```python
from build123d import *

# Parameters (mm, degrees)
BOSS_EXTRUDE2_DEPTH = 6.35
CUT_EXTRUDE1_DEPTH  = 7.3500001
BOSS_EXTRUDE3_DEPTH = 6.35
SKETCH10_R          = 3.96875
CUT_EXTRUDE2_DEPTH  = 7.35
SKETCH11_R          = 9.525
CUT_EXTRUDE4_DEPTH  = 7.35
BOSS_EXTRUDE4_DEPTH = 6.35
SKETCH13_R          = 1.75
CUT_EXTRUDE5_DEPTH  = 7.35
LPATTERN1_COUNT     = 2
LPATTERN1_PITCH     = 64
SKETCH14_R          = 2.54
CUT_EXTRUDE6_DEPTH  = 7.35
SKETCH15_R          = 1.75
CUT_EXTRUDE7_DEPTH  = 7.35
SKETCH16_R          = 1.75
CUT_EXTRUDE8_DEPTH  = 7.35
SKETCH17_R          = 1.75
CUT_EXTRUDE9_DEPTH  = 7.35
SKETCH19_R          = 3.96875
CUT_EXTRUDE11_DEPTH = 7.35
SKETCH21_R          = 2.54
CUT_EXTRUDE12_DEPTH = 7.35
SKETCH22_R          = 3.175
CUT_EXTRUDE13_DEPTH = 7.35
SKETCH23_R          = 3.96875
CUT_EXTRUDE14_DEPTH = 7.35
SKETCH24_R          = 4.285761756
SKETCH24_R_2        = 5.640780493
BOSS_EXTRUDE5_DEPTH = 6.35
CUT_EXTRUDE15_DEPTH = 7.35
FILLET1_R           = 3.175


with BuildPart() as part:
    # Sketch6 → Boss-Extrude2 (new body)
    with BuildSketch(Plane.XY):
        with BuildLine():
            Line((-68.006850091, -76.67090114), (-109.486767671, -48.656527855))
            Line((-109.486767671, -48.656527855), (-118.371760678, -61.812230963))
            Line((-118.371760678, -61.812230963), (18.447551645, -154.216158235))
            Line((18.447551645, -154.216158235), (135.729459338, 19.43912279))
            Line((135.729459338, 19.43912279), (-1.089852986, 111.843050063))
            Line((-1.089852986, 111.843050063), (-73.946795643, 3.966284577))
            Line((-73.946795643, 3.966284577), (-56.624438948, -7.732749433))
            ThreePointArc((-56.624438948, -7.732749433), (-43.058385537, 37.577891571), (0, 57.15))
            ThreePointArc((0, 57.15), (56.404848571, 31.095576642), (70.829334649, -29.338471048))
            add(Edge.make_bspline(
                [(70.829334649, -29.338471048), (70.811686062, -29.418295928), (70.776015112, -29.578104383), (70.713320217, -29.85478305), (70.619021771, -30.262929245), (70.501052001, -30.762086912), (70.364034474, -31.322191481), (70.199318515, -31.970958926), (70.000453855, -32.723919765), (69.795103485, -33.469783355), (69.582015398, -34.214296028), (69.361377803, -34.956693289), (69.133257682, -35.696762218), (68.838782679, -36.61892651), (68.470566207, -37.720710028), (68.019498024, -38.998776477), (67.474836154, -40.448808619), (66.901337925, -41.887676852), (66.299328392, -43.31485223), (65.669141732, -44.729810424), (65.011119088, -46.132040323), (64.325609411, -47.52103904), (63.612968547, -48.896314904), (62.87355937, -50.257385735), (62.107751613, -51.603779381), (61.315921169, -52.935034173), (60.49845004, -54.250698756), (59.655726138, -55.550331897), (58.571247582, -57.154294757), (57.220953058, -59.045283389), (55.576035723, -61.200397094), (53.604026134, -63.590264702), (51.54329346, -65.904053004), (49.39728314, -68.138962994), (47.169496434, -70.29235602), (44.863486103, -72.361752995), (42.482847363, -74.344831806), (40.031215607, -76.239428526), (36.882516177, -78.494556171), (32.976808929, -81.016011003), (28.250788286, -83.68089187), (21.41551215, -86.919136497), (14.30829026, -89.526654921), (6.996956895, -91.488176442), (-0.451922312, -92.797413176), (-6.61686174, -93.456358442), (-12.81195397, -93.702029749), (-19.009644204, -93.537285056), (-25.183124422, -92.966685286), (-31.306438312, -91.996382122), (-36.598524037, -90.804323442), (-41.072542301, -89.543185606), (-44.752319298, -88.33589156), (-47.664184976, -87.27761875), (-50.541347258, -86.128353728), (-53.381128552, -84.889612663), (-56.180924218, -83.562977818), (-58.593536599, -82.326710176), (-60.633378351, -81.214215821), (-62.313751085, -80.252471782), (-63.646071553, -79.462491566), (-64.966093336, -78.652178853), (-66.222359154, -77.854259082), (-67.143044791, -77.250601571), (-67.736251212, -76.85365602), (-68.006850091, -76.67090114)],
                knots=[0.071020771, 0.071020771, 0.071020771, 0.071020771, 0.071020771, 0.072848477, 0.074676184, 0.07650389, 0.078331597, 0.08198701, 0.085642423, 0.089297836, 0.092953249, 0.096608662, 0.100264075, 0.103919488, 0.107574901, 0.114885727, 0.122196554, 0.12950738, 0.136818214, 0.144129048, 0.151439882, 0.158750716, 0.166061558, 0.173372401, 0.180683243, 0.187994085, 0.195304924, 0.202615763, 0.209926602, 0.217237441, 0.231859103, 0.246480766, 0.261102426, 0.275724085, 0.290345754, 0.304967424, 0.319589099, 0.334210774, 0.348832457, 0.36345414, 0.392697464, 0.421940789, 0.451184112, 0.506140643, 0.535383973, 0.564627303, 0.593870641, 0.623113979, 0.652357319, 0.68160066, 0.710843985, 0.740087309, 0.754708984, 0.769330659, 0.783952333, 0.798574008, 0.813195669, 0.82781733, 0.842438991, 0.849749821, 0.857060652, 0.86437149, 0.871682327, 0.878993165, 0.885158103, 0.885158103, 0.885158103, 0.885158103, 0.885158103], degree=4))
        make_face()
    extrude(amount=BOSS_EXTRUDE2_DEPTH)

    # Sketch8 → Cut-Extrude1 (cut, through all)
    with BuildSketch(Plane.XY.offset(6.35)):
        Polygon((-71.011229489, -93.798205788), (-53.378672597, -90.381637707), (-42.854110111, -97.489632113), (-39.43754203, -115.122189004), align=None)
    extrude(amount=-CUT_EXTRUDE1_DEPTH, mode=Mode.SUBTRACT)

    # Sketch9 → Boss-Extrude3 (add, through all)
    with BuildSketch(Plane.XY.offset(6.35)):
        Polygon((-1.089852986, 111.843050063), (-109.486767671, -48.656527855), (27.332544652, -141.060455127), (135.729459338, 19.43912279), align=None)
    extrude(amount=-BOSS_EXTRUDE3_DEPTH)

    # Sketch10 → Cut-Extrude2 (cut, through all)
    with BuildSketch(Plane.XY.offset(6.35)):
        with Locations((4.996496209, -84.796642912)):
            Circle(SKETCH10_R)
        with Locations((40.816310536, -31.759477627)):
            Circle(SKETCH10_R)
        with Locations((76.636124864, 21.277687659)):
            Circle(SKETCH10_R)
        with Locations((-45.295165913, -45.214466102)):
            Circle(SKETCH10_R)
    extrude(amount=-CUT_EXTRUDE2_DEPTH, mode=Mode.SUBTRACT)

    # Sketch11 → Cut-Extrude4 (cut, through all)
    with BuildSketch(Plane.XY.offset(6.35)):
        Circle(SKETCH11_R)
    extrude(amount=-CUT_EXTRUDE4_DEPTH, mode=Mode.SUBTRACT)

    # Sketch12 → Boss-Extrude4 (add, through all)
    with BuildSketch(Plane.XY.offset(6.35)):
        Polygon((135.729459338, 19.43912279), (67.319803176, 65.641086427), (88.643786393, 97.214773886), (157.053442554, 51.01281025), align=None)
    extrude(amount=-BOSS_EXTRUDE4_DEPTH)

    # Sketch13 → Cut-Extrude5 (cut, through all)
    with BuildSketch(Plane.XY.offset(6.35)):
        with Locations((94.899221836, -29.671127724)):
            Circle(SKETCH13_R)
    cut_extrude5 = extrude(amount=-CUT_EXTRUDE5_DEPTH, mode=Mode.SUBTRACT)

    # LPattern1: Cut-Extrude5 ×2
    with Locations(*[Vector(-0.559684599, -0.828705708, 0) * (i * LPATTERN1_PITCH) for i in range(1, LPATTERN1_COUNT)]):
        add(cut_extrude5, mode=Mode.SUBTRACT)

    # Sketch14 → Cut-Extrude6 (cut, through all)
    with BuildSketch(Plane.XY.offset(6.35)):
        with Locations((71.72703343, -52.635713164)):
            Circle(SKETCH14_R)
        with Locations((35.907219102, -105.67287845)):
            Circle(SKETCH14_R)
        with Locations((115.740620068, 63.589229581)):
            Circle(SKETCH14_R)
    extrude(amount=-CUT_EXTRUDE6_DEPTH, mode=Mode.SUBTRACT)

    # Sketch15 → Cut-Extrude7 (cut, through all)
    with BuildSketch(Plane.XY.offset(6.35)):
        with Locations((-105.147343009, -59.249804902)):
            Circle(SKETCH15_R)
        with Locations((15.885125585, -140.991740566)):
            Circle(SKETCH15_R)
        with Locations((1.472573075, 98.618632394)):
            Circle(SKETCH15_R)
    extrude(amount=-CUT_EXTRUDE7_DEPTH, mode=Mode.SUBTRACT)

    # Sketch16 → Cut-Extrude8 (cut, through all)
    with BuildSketch(Plane.XY.offset(6.35)):
        with Locations((92.060354474, 79.582216994)):
            Circle(SKETCH16_R)
        with Locations((139.420885662, 47.596242169)):
            Circle(SKETCH16_R)
    extrude(amount=-CUT_EXTRUDE8_DEPTH, mode=Mode.SUBTRACT)

    # Sketch17 → Cut-Extrude9 (cut, through all)
    with BuildSketch(Plane.XY.offset(6.35)):
        with Locations((-26.311406216, 17.769986014)):
            Circle(SKETCH17_R)
        with Locations((17.769986014, 26.311406216)):
            Circle(SKETCH17_R)
    extrude(amount=-CUT_EXTRUDE9_DEPTH, mode=Mode.SUBTRACT)

    # Sketch19 → Cut-Extrude11 (cut, through all)
    with BuildSketch(Plane.XY.offset(6.35)):
        with Locations((-65.680233685, -85.904783923)):
            Circle(SKETCH19_R)
    extrude(amount=-CUT_EXTRUDE11_DEPTH, mode=Mode.SUBTRACT)

    # Sketch21 → Cut-Extrude12 (cut, through all)
    with BuildSketch(Plane.XY.offset(6.35)):
        with Locations((-13.666272317, 70.530227577)):
            Circle(SKETCH21_R)
        with Locations((26.00698069, 78.217505758)):
            Circle(SKETCH21_R)
        with Locations((-86.729358658, -71.688795112)):
            Circle(SKETCH21_R)
        with Locations((-8.64928203, -120.590613931)):
            Circle(SKETCH21_R)
    extrude(amount=-CUT_EXTRUDE12_DEPTH, mode=Mode.SUBTRACT)

    # Sketch22 → Cut-Extrude13 (cut, through all)
    with BuildSketch(Plane.XY.offset(6.35)):
        with Locations((-26.311406216, 17.769986014)):
            Circle(SKETCH22_R)
        with Locations((17.769986014, 26.311406216)):
            Circle(SKETCH22_R)
    extrude(amount=-CUT_EXTRUDE13_DEPTH, mode=Mode.SUBTRACT)

    # Sketch23 → Cut-Extrude14 (cut, through all)
    with BuildSketch(Plane.XY.offset(6.35)):
        with Locations((-105.147343009, -59.249804902)):
            Circle(SKETCH23_R)
    extrude(amount=-CUT_EXTRUDE14_DEPTH, mode=Mode.SUBTRACT)

    # Sketch24 → Boss-Extrude5 (add, through all)
    with BuildSketch(Plane.XY.offset(6.35)):
        with Locations((-86.729358658, -71.688795112)):
            Circle(SKETCH24_R)
        with Locations((-65.680233685, -85.904783923)):
            Circle(SKETCH24_R_2)
    extrude(amount=-BOSS_EXTRUDE5_DEPTH)

    # Sketch25 → Cut-Extrude15 (cut, through all)
    with BuildSketch(Plane.XY.offset(6.35)):
        Polygon((85.800588631, 93.004948891), (87.167215863, 85.951926135), (71.529628171, 62.797888664), (67.319803176, 65.641086427), align=None)
    extrude(amount=-CUT_EXTRUDE15_DEPTH, mode=Mode.SUBTRACT)

    # Fillet1
    fillet1_edges = [part.edges().sort_by_distance(p)[0] for p in [
        (-1.089852986, 111.843050063, 3.175),
        (18.447551645, -154.216158235, 3.175),
        (-118.371760678, -61.812230963, 3.175),
        (85.800588631, 93.004948891, 3.175),
        (87.167215863, 85.951926135, 3.175),
        (71.529628171, 62.797888664, 3.175),
        (-39.43754203, -115.122189004, 3.175),
        (-71.011229489, -93.798205788, 3.175),
        (-53.378672597, -90.381637707, 3.175),
        (-42.854110111, -97.489632113, 3.175),
        (157.053442554, 51.01281025, 3.175),
        (88.643786393, 97.214773886, 3.175),
    ]]
    fillet(fillet1_edges, radius=FILLET1_R)


solid = part.part
```
The listing builds one solid part. Answer for the finished solid, in the listing's coordinates (mm). A direction names the side the tool comes from. Give positions to 0.01 mm unless a question says otherwise; leave off trailing zeros. Order: outer loops, then holes, each group sorted by start corner. A loop starts at its lowest first (then second) coordinate and runs counter-clockwise, first axis right, second up.
Item 1: For a pull along Y with two mould halves and no side action, classify faces 3 (the face through (-28.65, 19.92, 3.22)), 4 (the face through (-48.17, -93.9, 3.22)), 5 (the face through (21, -19, 6.35)) as pulls with the +Y half, pulls with the -Y half, needs draft (parallel to the pull), parting line crosses it, or undercut.
From the geometry:
face 3: undercut
face 4: pulls with the -Y half
face 5: needs draft
Item 2: Find the intervals of material crossed by probe 1 along X at (y, z) = (77, 3.25); probe 2 along X at (y, z) = (65.5, 4.5); probe 3 along Y at (x, z) = (0, 3.5) (3 decimals), in increasing order.
From the geometry:
probe 1: x = -24.62 to 23.78, 28.24 to 50.5, 81.12 to 118.58
probe 2: x = -32.39 to 67.53, 73.35 to 114.07, 117.41 to 135.6
probe 3: y = -141.757 to -9.525, 9.525 to 97.673, 99.564 to 110.601
Item 3: The part is cut by section C-C, the plane y = -72.5. Give the vertices of the cut face in (x, z).
From the geometry:
outline: (-102.55, 0) - (73.64, 0) - (73.64, 6.35) - (-102.55, 6.35) - close
Item 4: The part is cut by section A-A, the plane y = 0. Give the vertices of the cut face in (x, z) (3 decimals), and give its area (3 significant figures).
From the geometry:
outline: (-76.626, 0) - (-9.525, 0) - (-9.525, 6.35) - (-76.626, 6.35) - close; (9.525, 0) - (122.601, 0) - (122.601, 6.35) - (9.525, 6.35) - close
area: 1,140 mm2
Item 5: The part is cut by section B-B, the plane z = 2.75. Count the separate pieces of the cut face and the enclosed holes in it, and give its area (3 significant figures).
From the geometry:
separate pieces: 1
enclosed holes: 20
area: 36,500 mm2
Item 6: The part is cut by section D-D, the plane x = -78. Give the vertices of the cut face in (y, z).
From the geometry:
outline: (-89.08, 0) - (-2.04, 0) - (-2.04, 6.35) - (-89.08, 6.35) - close
Item 7: Which of the six approach directions +Z, -Z, +X, -X, +Y, -Y give full straight-line access (tool end or side, diameter ignored) to faces 1 (the face through (-62.3, -92.11, 3.22)), 2 (the face through (39.956, -35.634, 3.219))?
From the geometry:
face 1: +Z, -Z, -Y
face 2: +Z, -Z
Item 8: Given pin 1 Ø5.5 at (x, y) = (94.9, -29.67) entering from -Z; pin 2 Ø6.5 at (x, y) = (5, -84.8) entering from -Z; pin 3 Ø2 at (y, z) = (-27.5, 4.5) entering from +X; pin 4 Ø1.5 at (y, z) = (60, 2) entering from -X, each flat-ended and moving along its own axis, determine where each tip first touches the part or whether it passes through.
From the geometry:
pin 1: stops at z = 0
pin 2: passes through
pin 3: stops at x = 104.7
pin 4: stops at x = -36.61
